The listing builds one solid part. Answer for the finished solid, in the listing's coordinates (mm). A direction names the side the tool comes from. Give positions to 0.01 mm unless a question says otherwise; leave off trailing zeros. Loops run counter-clockwise (first coordinate to the right, second up) from the corner with the lowest first, then second, coordinate; pieces in that order, holes last.
Item 1: Section B-B, the plane z = -0.25 is taken. Give the vertices of the cut face in (x, y).
Item 2: The mould has two halves that part along Z. Classify faces 4 (the face through (6, 1, 8)), 5 (the face through (5.754, 0.33, 7.493)), 6 (the face through (3, -3, 0)), 7 (the face through (2.96, 4.38, 8.43)): pulls with the +Z half, pulls with the -Z half, needs draft (parallel to the pull), parting line crosses it, or undercut.
Item 3: Consider line 1 along Z through (x, y) = (0.3, 1.25); line 2 along X through (y, z) = (-5, -5); line 3 along Z through (x, y) = (1.9, 0). Determine where each line is inside the solid, lowest interval first.
Item 4: Section D-D, the plane y = -4.5 is taken. Give the vertices of the cut face in (x, z).
Item 5: Section A-A, the plane y = 0 is taken. Give the vertices of the cut face in (x, z).
Item 6: Section C-C, the plane x = 2.35 is taken. Give the vertices of the cut face in (y, z).
Item 7: A tool of negligible diameter and unlimited length cuts with its end or side. For faces 1 (the face through (5.754, -3.905, 0.867)), 2 (the face through (0.246, -3.905, -0.867)), 3 (the face through (0, 1, 3)), from which of +Z, -Z, +X, -X, +Y, -Y can it reach the whole face along a straight path? Write none if from no direction.
Item 8: Each of these flat-tipped pins is pushed along its axis until it touches: pin 1 Ø1 at (x, z) = (4.5, 6.5) entering from +Y; pin 2 Ø7.5 at (y, z) = (-0.5, -2.5) entering from +X; pin 3 Ø3 at (x, y) = (4, 3.5) entering from -Z. Where does it stop, or does it pass through?
Autodesk Inventor part; units mm, degrees
ref_plane "YZ Plane" through (0, 0, 0) normal (1, 0, 0) x (0, 1, 0)
ref_plane "XZ Plane" through (0, 0, 0) normal (0, 1, 0) x (-1, 0, 0)
ref_plane "XY Plane" through (0, 0, 0) normal (0, 0, 1) x (1, 0, 0)
sketch "スケッチ1" plane through (0, 0, 0) normal (1, 0, 0) x (0, 1, 0)
  circle A0 centre (0, 0) radius 3
  circle A1 centre (0, 0) radius 9.5
  dimension "d0" = 6
  dimension "d1" = 19
extrude "押し出し1" add sketch "スケッチ1" along normal blind 6
sketch "スケッチ2" plane through (6, 0, 0) normal (1, 0, 0) x (0, 0, -1)
  circle A0 centre (0, 0) radius 4
  circle A1 centre (0, 0) radius 7.5
  dimension "d4" = 8
  dimension "d5" = 15
extrude "押し出し2" cut sketch "スケッチ2" against normal blind 0.5
sketch "スケッチ3" plane through (0, 0, 0) normal (-1, 0, 0) x (0, 0, 1)
  circle A0 centre (0, 0) radius 4
  circle A1 centre (0, 0) radius 7.5
  dimension "d8" = 8
  dimension "d9" = 15
extrude "押し出し3" cut sketch "スケッチ3" against normal blind 0.5
properties part number "Bearing_626ZZ" material "ステンレス鋼"
Worked answers:
1. outline: (0, -9.5) - (6, -9.5) - (6, -7.5) - (5.5, -7.5) - (5.5, -3.99) - (6, -3.99) - (6, -2.99) - (0, -2.99) - (0, -3.99) - (0.5, -3.99) - (0.5, -7.5) - (0, -7.5) - close; (0, 2.99) - (6, 2.99) - (6, 3.99) - (5.5, 3.99) - (5.5, 7.5) - (6, 7.5) - (6, 9.5) - (0, 9.5) - (0, 7.5) - (0.5, 7.5) - (0.5, 3.99) - (0, 3.99) - close
2. face 4: needs draft
2. face 5: undercut
2. face 6: undercut
2. face 7: parting line crosses it
3. line 1: z = -9.42 to -7.4, -3.8 to -2.73, 2.73 to 3.8, 7.4 to 9.42
3. line 2: x = 0.5 to 5.5
3. line 3: z = -9.5 to -3, 3 to 9.5
4. outline: (0, -8.37) - (6, -8.37) - (6, -6) - (5.5, -6) - (5.5, 6) - (6, 6) - (6, 8.37) - (0, 8.37) - (0, 6) - (0.5, 6) - (0.5, -6) - (0, -6) - close
5. outline: (0, -9.5) - (6, -9.5) - (6, -7.5) - (5.5, -7.5) - (5.5, -4) - (6, -4) - (6, -3) - (0, -3) - (0, -4) - (0.5, -4) - (0.5, -7.5) - (0, -7.5) - close; (0, 3) - (6, 3) - (6, 4) - (5.5, 4) - (5.5, 7.5) - (6, 7.5) - (6, 9.5) - (0, 9.5) - (0, 7.5) - (0.5, 7.5) - (0.5, 4) - (0, 4) - close
6. outline: circle Ø19 at (0, 0); hole circle Ø6 at (0, 0)
7. face 1: +X
7. face 2: -X
7. face 3: +Z, -Z, -X, +Y, -Y
8. pin 1: stops at y = 7.37
8. pin 2: stops at x = 6
8. pin 3: stops at z = -9.29
